```python
from build123d import *

# Parameters (mm, degrees)
F1_DEPTH = 5
F2_R     = 1
F4_R     = 11
F5_DEPTH = 12
F6_SIZE  = 0.5
F7_R     = 5.5
F8_DEPTH = 17.001


with BuildPart() as f1:
    # F0 (on Top) → F1 (new body)
    with BuildSketch(Plane.XY):
        Polygon((6.5, 11.25833), (-6.5, 11.25833), (-13, 0), (-6.5, -11.25833), (6.5, -11.25833), (13, 0), align=None)
    extrude(amount=-F1_DEPTH)

    # F2
    f2_edges = [f1.edges().sort_by_distance(p)[0] for p in [
        (6.5, -11.25833, -2.5),
        (-6.5, -11.25833, -2.5),
        (-13, 0, -2.5),
        (13, 0, -2.5),
        (6.5, 11.25833, -2.5),
        (-6.5, 11.25833, -2.5),
    ]]
    fillet(f2_edges, radius=F2_R)

    # F4 (on offset) → F5 (join)
    with BuildSketch(Plane(origin=(0, 0, -5), x_dir=(1, 0, 0), z_dir=(0, 0, -1))):
        Circle(F4_R)
    extrude(amount=F5_DEPTH)

    # F6
    f6_edges = [f1.edges().sort_by_distance(p)[0] for p in [
        (-11, 0, -17),
    ]]
    chamfer(f6_edges, length=F6_SIZE)

    # F7 (on face) → F8 (cut, through all)
    with BuildSketch(Plane(origin=(0, 0, -17), x_dir=(1, 0, 0), z_dir=(0, 0, -1))):
        Circle(F7_R)
    extrude(amount=-F8_DEPTH, mode=Mode.SUBTRACT)


solid = f1.part
```
Here's how the part is built. I have some questions about the finished solid (model axes, mm). A direction names the side the tool comes from. Coordinates: 2 decimals unless noted, no trailing zeros. Write each loop counter-clockwise with the first axis right and the second up, starting at its lowest first coordinate (ties: lowest second). Pieces come first, ordered by that corner, then holes. Notation, with made-up numbers: M -13,21 L -6,21 A17 ccw -6,32 Z; hole C 80,89.25 d3. An arc over 180 degrees is marked long. Answer as CSV lines item,"result". Start each with the question number.
Q1. Suppose I cut it at B-B, the plane y = 0. List the corners of the cut face in (x, z) for me.
Q2. If we mould it in two halves opening along Y, with no side actions, what happens to faces 1 (the cylindrical face through (-12.845, 0.007, -2.535)), 2 (the cylindrical face through (6.416, -11.128, -2.535)), 3 (the flat face through (6, 0, 0)), 4 (the cylindrical face through (-1.19, 5.37, -8.62))? For each: pulls with the +Y half, pulls with the -Y half, needs draft (parallel to the pull), parting line crosses it, or undercut.
Q3. Suppose I cut it at D-D, the plane z = -6.25. List the corners of the cut face in (x, y) for me.
Q4. Suppose I cut it at C-C, the plane z = -2.5. List the corners of the cut face in (x, y) for me.
Q5. I need wall thicknesses on probe 1 along X at (y, z) = (0, -12); probe 2 along Y at (x, z) = (0, -3.75). Which ranges of each line are inside material? Lowest first, please. Write a range as [from, to].
Q6. Will these pins go through, and if not, where does the flat tip stop? pin 1 Ø1.5 at (y, z) = (5.5, -11.5) entering from -X; pin 2 Ø8 at (x, z) = (2, -15) entering from +Y; pin 3 Ø2 at (y, z) = (2, -7) entering from -X.
Q7. Suppose I cut it at A-A, the plane x = 0. List the corners of the cut face in (y, z) for me.
Q8. For faces 5 (the flat face through (9.79, 5.56, -2.46)), 6 (the flat face through (-11, 3, -5)), which set-ups out of +Z, -Z, +X, -X, +Y, -Y let a thin tool reach every point of the face, with its end or its side?
Entries:
1,outline,"M -12.85,-5 L -11,-5 L -11,-16.5 L -10.5,-17 L -5.5,-17 L -5.5,0 L -12.85,0 Z; M 5.5,-17 L 10.5,-17 L 11,-16.5 L 11,-5 L 12.85,-5 L 12.85,0 L 5.5,0 Z"
2,face 1,"parting line crosses it"
2,face 2,"pulls with the -Y half"
2,face 3,"needs draft"
2,face 4,"undercut"
3,outline,"C 0,0 d22; hole C 0,0 d11"
4,outline,"M -12.71,-0.5 L -6.79,-10.76 A1 ccw -5.92,-11.26 L 5.92,-11.26 A1 ccw 6.79,-10.76 L 12.71,-0.5 A1 ccw 12.71,0.5 L 6.79,10.76 A1 ccw 5.92,11.26 L -5.92,11.26 A1 ccw -6.79,10.76 L -12.71,0.5 A1 ccw Z; hole C 0,0 d11"
5,probe 1,"x = [-11, -5.5], [5.5, 11]"
5,probe 2,"y = [-11.26, -5.5], [5.5, 11.26]"
6,pin 1,"stops at x = -9.92"
6,pin 2,"stops at y = 11"
6,pin 3,"stops at x = -10.95"
7,outline,"M -11.26,-5 L -11,-5 L -11,-16.5 L -10.5,-17 L -5.5,-17 L -5.5,0 L -11.26,0 Z; M 5.5,-17 L 10.5,-17 L 11,-16.5 L 11,-5 L 11.26,-5 L 11.26,0 L 5.5,0 Z"
8,face 5,"+Z, -Z, +X, +Y"
8,face 6,"-Z"
